Can you work these out from the drawing? Everything is in mm from the part's minimum corner. Coordinates: 2 decimals unless noted, no trailing zeros. Loops run counter-clockwise (first coordinate to the right, second up) from the corner with the lowest first, then second, coordinate; pieces in that order, holes last. Notation, with made-up numbers: (-10, 83.5) -> (19, 83.5) arc R16 cw to (19, 107.5) -> close; hole circle Ø4 at (28.25, 87). An arc over 180 degrees is marked (long way). Use one line per item in the form item = value. Start each with the question number.
(1) Imagine slicing it at D-D (y = 28). List the corners of the cut face in (x, z) for me.
(2) Imagine slicing it at B-B (y = 21.5). List the corners of the cut face in (x, z) for me.
(3) Imagine slicing it at C-C (x = 39.5). List the corners of the cut face in (y, z) for me, plus the area to 3 significant figures.
(4) I need wall thicknesses on line 1 (Y direction, x = 38.5, z = 3.5); line 2 (Y direction, x = 40, z = 2.75); line 3 (X direction, y = 25.5, z = 9) (1 decimal). Which ranges of each line are inside material? Lowest first, please. Write a range as [from, to].
(5) Imagine slicing it at A-A (z = 7.75). List the corners of the cut face in (x, y) for me.
(6) Thinking about a two-plate mould opening in Z: for the marked faces 1, 2 and 3, which applies, released by +Z, released by -Z, zero draft, split by the parting line, or undercut?
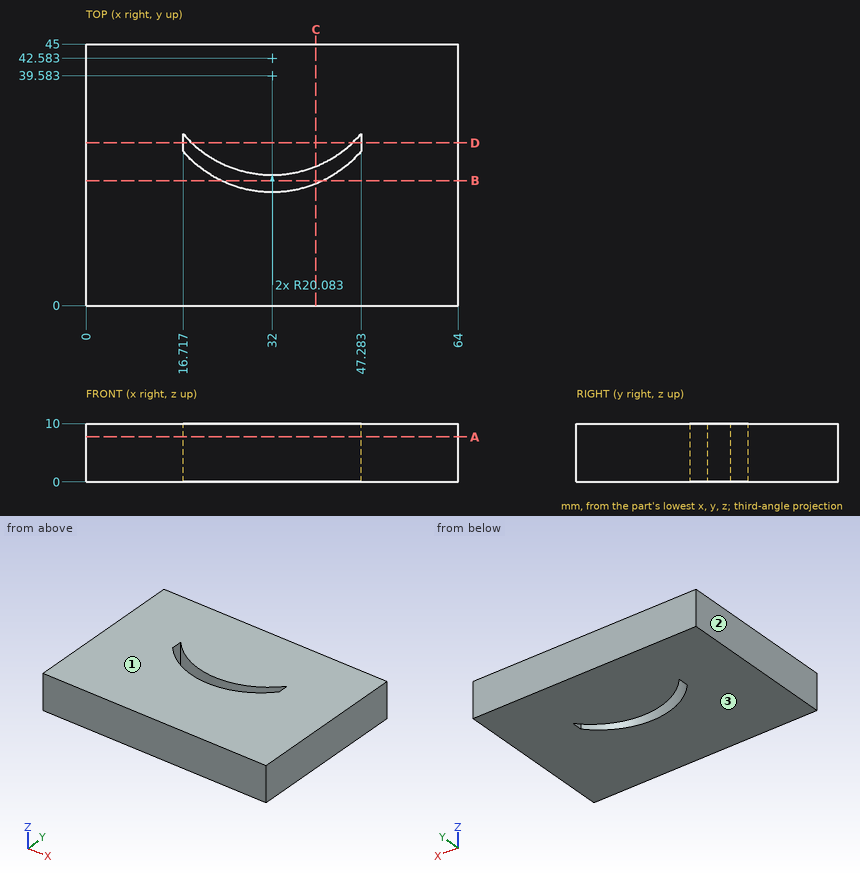
Worked out:
q1.outline = (0, 0) -> (16.72, 0) -> (16.72, 10) -> (0, 10) -> close; (18.19, 0) -> (45.81, 0) -> (45.81, 10) -> (18.19, 10) -> close; (47.28, 0) -> (64, 0) -> (64, 10) -> (47.28, 10) -> close
q2.outline = (0, 0) -> (23.26, 0) -> (23.26, 10) -> (0, 10) -> close; (40.74, 0) -> (64, 0) -> (64, 10) -> (40.74, 10) -> close
q3.outline = (0, 0) -> (20.95, 0) -> (20.95, 10) -> (0, 10) -> close; (23.95, 0) -> (45, 0) -> (45, 10) -> (23.95, 10) -> close
q3.area = 420 mm2
q4.line_1 = [0, 20.58], [23.58, 45]
q4.line_2 = [0, 21.16], [24.16, 45]
q4.line_3 = [0, 17.7], [21.4, 42.6], [46.3, 64]
q5.outline = (0, 0) -> (64, 0) -> (64, 45) -> (0, 45) -> close; hole (16.72, 26.55) arc R20.08 ccw to (47.28, 26.55) -> (47.28, 29.55) arc R20.08 cw to (16.72, 29.55) -> close
q6.face_1 = released by +Z
q6.face_2 = zero draft
q6.face_3 = released by -Z
